```python
from build123d import *

# Parameters (mm, degrees)
F1_DEPTH = 25


with BuildPart() as f1:
    # F0 (on Top) → F1 (new body)
    with BuildSketch(Plane.XY):
        with BuildLine():
            ThreePointArc((24.8701038765, -6.5218529704), (25.4999256036, -3.2879214113), (25.7110216249, 0))
            ThreePointArc((25.7110216249, 0), (25.1255094172, 5.4557684631), (23.3956403104, 10.6630505701))
            ThreePointArc((23.3956403104, 10.6630505701), (17.2285716474, 19.0848880527), (8.2217665775, 24.3610177813))
            ThreePointArc((8.2217665775, 24.3610177813), (-0.1258474148, 25.7107136311), (-8.459848903, 24.2793655093))
            ThreePointArc((-8.459848903, 24.2793655093), (-17.3538464261, 18.9710476046), (-23.4315262789, 10.5839599978))
            ThreePointArc((-23.4315262789, 10.5839599978), (-25.5543270236, 2.8342553459), (-25.1812828872, -5.1922658973))
            ThreePointArc((-25.1812828872, -5.1922658973), (-19.3520995784, -16.9278727223), (-8.4963727751, -24.2666083881))
            ThreePointArc((-8.4963727751, -24.2666083881), (-1.0796944371, -25.6883415758), (6.430127649, -24.8939770108))
            ThreePointArc((6.430127649, -24.8939770108), (18.146896672, -18.2139170463), (24.8701038765, -6.5218529704))
        make_face()
        with BuildLine():
            ThreePointArc((23.3956403104, 10.6630505701), (25.1255094172, 5.4557684631), (25.7110216249, 0))
            ThreePointArc((25.7110216249, 0), (25.4999256036, -3.2879214113), (24.8701038765, -6.5218529704))
            Line((24.8701038765, -6.5218529704), (73.9221572876, 0))
            Line((73.9221572876, 0), (23.3956403104, 10.6630505701))
        make_face()
        with BuildLine():
            ThreePointArc((-8.459848903, 24.2793655093), (-0.1258474148, 25.7107136311), (8.2217665775, 24.3610177813))
            Line((8.2217665775, 24.3610177813), (0, 74.7051164508))
            Line((0, 74.7051164508), (-8.459848903, 24.2793655093))
        make_face()
        with BuildLine():
            ThreePointArc((-25.1812828872, -5.1922658973), (-25.5543270236, 2.8342553459), (-23.4315262789, 10.5839599978))
            Line((-23.4315262789, 10.5839599978), (-76.5798836946, 3.3824506681))
            Line((-76.5798836946, 3.3824506681), (-25.1812828872, -5.1922658973))
        make_face()
    extrude(amount=F1_DEPTH)


solid = f1.part
```
The model under review builds one solid part; all positions refer to its coordinate system, in mm. Round coordinates to 2 decimals unless told otherwise and drop trailing zeros. Order: outer loops, then holes, each group sorted by start corner. A loop starts at its lowest first (then second) coordinate and runs counter-clockwise, first axis right, second up.
Item 1: Add section A-A, the plane z = 4.5. State the section outline as (x, y) points, and give its area (3 significant figures).
Working result:
outline: (-76.58, 3.38) - (-25.18, -5.19) arc R25.71 ccw to (24.87, -6.52) - (73.92, 0) - (23.4, 10.66) arc R25.71 ccw to (8.22, 24.36) - (0, 74.71) - (-8.46, 24.28) arc R25.71 ccw to (-23.43, 10.58) - close
area: 3,290 mm2
Item 2: To check wall thickness, follow probe 1 along Y at (x, z) = (63.5, 24.25); probe 2 along Y at (x, z) = (35, 23.5) (3 decimals); probe 3 along X at (y, z) = (-17, 1.75). State the ranges of each line that lie inside material, in increasing order.
Working result:
probe 1: y = -1.39 to 2.2
probe 2: y = -5.175 to 8.214
probe 3: x = -19.29 to 19.29
Item 3: For pin 1 (2 mm diameter, centred on y = -12.5, z = 8, fed in from +X); pin 2 (6 mm diameter, centred on x = 37, z = 13, fed in from +Y); pin 3 (1.5 mm diameter, centred on y = -12, z = 11, fed in from -X); pin 4 (10 mm diameter, centred on x = 40.5, y = -13, fed in from +Z), all flat-tipped, find the tip position at first contact; note any pin that passes through.
Working result:
pin 1: stops at x = 23
pin 2: stops at y = 8.43
pin 3: stops at x = -23.12
pin 4: passes through
Item 4: Add section C-C, the plane x = 55.5. State the section outline as (y, z) points.
Working result:
outline: (-2.45, 0) - (3.89, 0) - (3.89, 25) - (-2.45, 25) - close
Item 5: Add section B-B, the plane y = 34.5. State the section outline as (x, z) points.
Working result:
outline: (-6.75, 0) - (6.57, 0) - (6.57, 25) - (-6.75, 25) - close
